Geometry check sheet. Reference: the model listing, model coordinates, mm. A direction names the side the tool comes from. Coordinates: 2 decimals unless noted, no trailing zeros. Write each loop counter-clockwise with the first axis right and the second up, starting at its lowest first coordinate (ties: lowest second). Pieces come first, ordered by that corner, then holes.
Autodesk Inventor part; units mm, degrees
ref_plane "YZ Plane" through (0, 0, 0) normal (1, 0, 0) x (0, 1, 0)
ref_plane "XZ Plane" through (0, 0, 0) normal (0, 1, 0) x (-1, 0, 0)
ref_plane "XY Plane" through (0, 0, 0) normal (0, 0, 1) x (1, 0, 0)
sketch "スケッチ1" plane through (0, 0, 0) normal (0, 1, 0) x (-1, 0, 0)
  line L0 (-17.5, 40) -> (-7.5, 40)
  line L1 (-7.5, 40) -> (-7.5, 30)
  line L2 (-7.5, 30) -> (-5, 27.5)
  line L3 (-5, 27.5) -> (5, 27.5)
  line L4 (5, 27.5) -> (7.5, 30)
  line L5 (7.5, 30) -> (7.5, 40)
  line L6 (7.5, 40) -> (17.5, 40)
  circle A0 centre (-12.5, 32.5) radius 1.5
  circle A1 centre (12.5, 32.5) radius 1.5
  line L7 (-17.5, 40) -> (-17.5, 27.5)
  line L8 (-17.5, 27.5) -> (-10, 20)
  line L9 (17.5, 40) -> (17.5, 27.5)
  line L10 (17.5, 27.5) -> (10, 20)
  line L11 (-10, 20) -> (-10, -40)
  line L12 (-10, -40) -> (-25.3553, -55.3553)
  line L13 (-11.2132, -69.4975) -> (10, -48.2843)
  line L14 (10, -48.2843) -> (10, 20)
  line L15 (0, 0) -> (47.4517, 0)
  line L16 (-21.8198, -58.8909) -> (-18.2843, -55.3553)
  line L17 (-11.2132, -62.4264) -> (-14.7487, -65.9619)
  arc A2 (-11.2132, -62.4264) -> (-18.2843, -55.3553) centre (-14.7487, -58.8909) ccw
  line L18 (-25.3553, -55.3553) -> (-21.8198, -58.8909)
  line L19 (-14.7487, -65.9619) -> (-11.2132, -69.4975)
  dimension "d2" = 10
  dimension "d3" = 135
  dimension "d4" = 45
  dimension "d6" = 15
  dimension "d7" = 2.5
  dimension "d8" = 10
  dimension "d9" = 10
  dimension "d10" = 10
  dimension "d11" = 10
  dimension "d12" = 90
  dimension "d15" = 25
  dimension "d16" = 5
  dimension "d17" = 20
  dimension "d18" = 7.5
  dimension "d19" = 7.5
  dimension "d20" = 5
  dimension "d21" = 60
  dimension "d22" = 20
  dimension "d23" = 135
  dimension "d24" = 10
  dimension "d27" = 20
  dimension "d28" = 20
  dimension "d29" = 90
  dimension "d31" = 3
  dimension "d33" = 10
  dimension "d35" = 10
  dimension "d37" = 5
  dimension "d38" = 5
  dimension "d39" = 5
  dimension "d40" = 30
extrude "押し出し2" add sketch "スケッチ1" along normal blind 2
sketch "スケッチ2" plane through (0, 2, 0) normal (0, 1, 0) x (1, 0, 0)
  line L0 (25.3553, 55.3553) -> (21.8198, 58.8909)
  arc A0 (11.2132, 62.4264) -> (18.2843, 55.3553) centre (14.7487, 58.8909) ccw
  circle A1 centre (19.6985, 53.9411) radius 1
  point P0 (0, 0)
  dimension "d48" = 5
  dimension "d49" = 7
  dimension "d50" = 2
hole "穴1" at (19.6985, 2, -53.9411) direction (0, -1, 0) diameter 2 end through all
pattern_circular "円形状パターン1" count 5 over 180 about axis through (14.7487, 0, -58.8909) along (0, -1, 0) of "穴1"
sketch "スケッチ3" plane through (0, 2, 0) normal (0, 1, 0) x (1, 0, 0)
  circle A0 centre (9.799, 63.8406) radius 1
  circle A1 centre (7.7487, 58.8909) radius 1
  circle A2 centre (9.799, 53.9411) radius 1
  circle A3 centre (14.7487, 51.8909) radius 1
  circle A4 centre (19.6985, 53.9411) radius 1
  circle A5 centre (-12.5, -32.5) radius 1.5
  circle A6 centre (12.5, -32.5) radius 1.5
  line L0 (7.5, -40) -> (17.5, -40)
  line L1 (17.5, -40) -> (17.5, -27.5)
  line L2 (17.5, -27.5) -> (10, -20)
  line L3 (10, -20) -> (10, 40)
  line L4 (10, 40) -> (25.3553, 55.3553)
  line L5 (25.3553, 55.3553) -> (21.8198, 58.8909)
  line L6 (21.8198, 58.8909) -> (18.2843, 55.3553)
  arc A7 (11.2132, 62.4264) -> (18.2843, 55.3553) centre (14.7487, 58.8909) ccw
  line L7 (11.2132, 62.4264) -> (14.7487, 65.9619)
  line L8 (14.7487, 65.9619) -> (11.2132, 69.4975)
  line L9 (11.2132, 69.4975) -> (-10, 48.2843)
  line L10 (-10, 48.2843) -> (-10, -20)
  line L11 (-10, -20) -> (-17.5, -27.5)
  line L12 (-17.5, -27.5) -> (-17.5, -40)
  line L13 (-17.5, -40) -> (-7.5, -40)
  line L14 (-7.5, -40) -> (-7.5, -30)
  line L15 (-7.5, -30) -> (-5, -27.5)
  line L16 (-5, -27.5) -> (5, -27.5)
  line L17 (5, -27.5) -> (7.5, -30)
  line L18 (7.5, -30) -> (7.5, -40)
  arc A8 (12.1605, 68.5501) -> (7.6777, 65.9619) centre (14.7487, 58.8909) ccw
  arc A9 (21.8198, 51.8198) -> (24.408, 56.3027) centre (14.7487, 58.8909) ccw
  point P0 (0, 0)
extrude "押し出し3" cut sketch "スケッチ3" against normal blind 2 contours L18 L17 L16 L15 L14 L13 L12 L11 L10 L9 A8 L8 L7 A7 L6 L5 A9 L4 L3 L2 L1 L0 keep common part
fillet "フィレット1" radius 2 4 edges at (14.7487, 1, -65.9619) (21.8198, 1, -58.8909) (24.408, 1, -56.3027) (12.1605, 1, -68.5501)
fillet "フィレット2" radius 2 4 edges at (-5, 1, 27.5) (-7.5, 1, 30) (5, 1, 27.5) (7.5, 1, 30)
properties part number "Arm_Link"
1. Sectioned sample at C-C, the plane z = -38. Record the boundary of the cut face in (x, y), and give its area (3 significant figures).
Computed values:
outline: (-10, 0) - (10, 0) - (10, 2) - (-10, 2) - close
area: 40.0 mm2
2. Sectioned sample at B-B, the plane z = 32.5. Record the boundary of the cut face in (x, y), and give its area (3 significant figures).
Computed values:
outline: (-17.5, 0) - (-14, 0) - (-14, 2) - (-17.5, 2) - close; (-11, 0) - (-7.5, 0) - (-7.5, 2) - (-11, 2) - close; (7.5, 0) - (11, 0) - (11, 2) - (7.5, 2) - close; (14, 0) - (17.5, 0) - (17.5, 2) - (14, 2) - close
area: 28.0 mm2
3. Draft check along X on faces 1 (the cylindrical face through (11.992, 0.986, -68.222)), 2 (the flat face through (-1.037, 0.986, -57.247)), 3 (the flat face through (7.5, 1, 35)). Enter one of: released by +X, released by -X, zero draft, split by the parting line, or undercut.
Computed values:
face 1: split by the parting line
face 2: released by -X
face 3: undercut
4. Thickness scan on line 1 along Z through (x, y) = (12.5, 1); line 2 along X through (y, z) = (1, -11); line 3 along Z through (x, y) = (-12.5, 0.95). Record the ranges inside material, lowest first.
Computed values:
line 1: z = -68.06 to -63.71, -54.43 to -42.5, 22.5 to 31, 34 to 40
line 2: x = -10 to 10
line 3: z = 22.5 to 31, 34 to 40
5. Sectioned sample at A-A, the plane x = -12.5. Record the boundary of the cut face in (y, z), and give its area (3 significant figures).
Computed values:
outline: (0, 22.5) - (2, 22.5) - (2, 31) - (0, 31) - close; (0, 34) - (2, 34) - (2, 40) - (0, 40) - close
area: 29.0 mm2
6. Sectioned sample at D-D, the plane y = 1.25. Give the number of separate pieces and of enclosed holes in the cut face, and give its area (3 significant figures).
Computed values:
separate pieces: 1
enclosed holes: 7
area: 2,140 mm2
7. Access from +Z, -Z, +X, -X, +Y, -Y to the whole of each face (thin tool, end or side, straight path). Record for faces 4 (the flat face through (19.36, 0.99, -56.43)), 5 (the flat face through (-7.5, 1, 35)), 6 (the flat face through (13, 1, 40)), 7 (the flat face through (16, 1, -46)).
Computed values:
face 4: -Z, +Y, -Y
face 5: +Z, +Y, -Y
face 6: +Z, +X, -X, +Y, -Y
face 7: +X, +Y, -Y
8. Gauge pin test, flat ends, axial feed: pin 1 Ø1 at (x, y) = (1, 1) entering from +Z; pin 2 Ø0.6 at (y, z) = (1, 2.5) entering from +X; pin 3 Ø0.6 at (y, z) = (1.5, -6.5) entering from -X. Record the tip position at first contact, or that the pin passes through.
Computed values:
pin 1: stops at z = 27.5
pin 2: stops at x = 10
pin 3: stops at x = -10
